Could you check a few things on this model? Use its own coordinates, in mm. A direction names the side the tool comes from. Coordinates: 2 decimals unless noted, no trailing zeros. Write each loop counter-clockwise with the first axis right and the second up, starting at its lowest first coordinate (ties: lowest second). Pieces come first, ordered by that corner, then holes.
```python
from build123d import *

# Parameters (mm, degrees)
BASE_FLANGE1_DEPTH = 711.2
SKETCH18_R         = 3.429
CUT_EXTRUDE1_DEPTH = 3.175
FILLET1_R          = 3.175
SKETCH20_R         = 3.175
CUT_EXTRUDE2_DEPTH = 3.175


# Sheet-metal steps are written as plain solids
with BuildPart() as part:
    # Sketch1 → Base-Flange1 (new body)
    with BuildSketch(Plane(origin=(0, 0, 0), x_dir=(0, 0, -1), z_dir=(1, 0, 0))):
        with BuildLine():
            Line((0, 0), (0, 31.75))
            ThreePointArc((0, 31.75), (1.859871939, 36.240128061), (6.35, 38.1))
            Line((6.35, 38.1), (38.1, 38.1))
            Line((38.1, 38.1), (38.1, 34.925))
            Line((38.1, 34.925), (6.35, 34.925))
            ThreePointArc((6.35, 34.925), (4.10493597, 33.99506403), (3.175, 31.75))
            Line((3.175, 31.75), (3.175, 0))
            Line((3.175, 0), (0, 0))
        make_face()
    extrude(amount=BASE_FLANGE1_DEPTH)

    # Sketch18 → Cut-Extrude1 (cut)
    with BuildSketch(Plane(origin=(0, 38.1, 0), x_dir=(1, 0, 0), z_dir=(0, 1, 0))):
        with Locations(Location((76.2, 22.225, 0), (0, 0, 270))):
            Circle(SKETCH18_R)
        with Locations(Location((355.6, 22.225, 0), (0, 0, 270))):
            Circle(SKETCH18_R)
        with Locations(Location((635, 22.225, 0), (0, 0, 270))):
            Circle(SKETCH18_R)
    extrude(amount=-CUT_EXTRUDE1_DEPTH, mode=Mode.SUBTRACT)

    # Fillet1
    fillet1_edges = [part.edges().sort_by_distance(p)[0] for p in [
        (711.2, 0, -1.5875),
        (0, 0, -1.5875),
        (711.2, 36.5125, -38.1),
        (0, 36.5125, -38.1),
    ]]
    fillet(fillet1_edges, radius=FILLET1_R)

    # Sketch20 → Cut-Extrude2 (cut)
    with BuildSketch(Plane.XY):
        with Locations((63.5, 12.7)):
            Circle(SKETCH20_R)
        with Locations((114.3, 12.7)):
            Circle(SKETCH20_R)
        with Locations((596.9, 12.7)):
            Circle(SKETCH20_R)
        with Locations((647.7, 12.7)):
            Circle(SKETCH20_R)
    extrude(amount=-CUT_EXTRUDE2_DEPTH, mode=Mode.SUBTRACT)


solid = part.part
```
1. I want a section at A-A on x = 338.5. Please give me the cut outline in (y, z) (3 decimals), plus the area to 3 significant figures.
Verdict:
outline: (0, -3.175) - (31.75, -3.175) arc R3.175 cw to (34.925, -6.35) - (34.925, -38.1) - (38.1, -38.1) - (38.1, -6.35) arc R6.35 ccw to (31.75, 0) - (0, 0) - close
area: 225 mm2
2. I want a section at B-B on y = 23. Please give me the cut outline in (x, z) (3 decimals).
Verdict:
outline: (0, -3.175) - (711.2, -3.175) - (711.2, 0) - (0, 0) - close
3. On a 3-axis mill with a long thin cutter (end or side, diameter ignored), from which of +Z, -Z, +X, -X, +Y, -Y can I reach the whole of each face in a straight line? I mean faces 1 (the face through (351, 16, -3.175)), 2 (the face through (0, 36, -12)). Say none if no direction works.
Verdict:
face 1: -Z, +X, -X, -Y
face 2: +Z, -Z, -X, +Y, -Y
4. Please list where these lines run through material, in increasing order: line 1 along X through (y, z) = (12, -2); line 2 along Y through (x, z) = (647.7, -1) (3 decimals); line 3 along Z through (x, y) = (646, 22) (3 decimals).
Verdict:
line 1: x = 0 to 60.4, 66.6 to 111.2, 117.4 to 593.8, 600 to 644.6, 650.8 to 711.2
line 2: y = 0 to 9.525, 15.875 to 35.171
line 3: z = -3.175 to 0
5. For pin 1 (2 mm diameter, centred on x = 474.5, y = 29.5, fed in from -Z) (3 decimals), with a flat end and sliding along its axis, tell me the tip position at first contact or that it passes through.
Verdict:
pin 1: stops at z = -3.175
